```python
from build123d import *

# Parameters (mm, degrees)
F0_R     = 50
F0_R_2   = 40
F1_DEPTH = 15
F2_R     = 50
F2_R_2   = 5
F3_DEPTH = 5
F4_R     = 5
F5_DEPTH = 40


with BuildPart() as f1:
    # F0 (on Front) → F1 (new body)
    with BuildSketch(Plane.XZ):
        Circle(F0_R)
        Circle(F0_R_2, mode=Mode.SUBTRACT)
    extrude(amount=F1_DEPTH)

    # F2 (on face) → F3 (join)
    with BuildSketch(Plane(origin=(0, 0, 0), x_dir=(-1, 0, 0), z_dir=(0, 1, 0))):
        Circle(F2_R)
        Circle(F2_R_2, mode=Mode.SUBTRACT)
    extrude(amount=F3_DEPTH)

    # F4 (on face) → F5 (join)
    with BuildSketch(Plane.XZ.offset(15)):
        with Locations((45, 0)):
            Circle(F4_R)
    extrude(amount=F5_DEPTH)


solid = f1.part
```
Build history of the part. All positions in model axes, mm. A direction names the side the tool comes from. Give positions to 0.01 mm unless a question says otherwise; leave off trailing zeros. Loops run counter-clockwise (first coordinate to the right, second up) from the corner with the lowest first, then second, coordinate; pieces in that order, holes last. Notation, with made-up numbers: (2, 63) - (33, 63) arc R18 ccw to (33, 97) - close; hole circle Ø8 at (31, 68.25). An arc over 180 degrees is marked (long way). Use a Markdown table: item, result.
(1) Band-saw the part on A-A (x = 0). Give the cut face in (y, z), and give its area (3 significant figures).
Taken from the geometry:
| item | result |
|---|---|
| outline | (-15, -50) - (5, -50) - (5, -5) - (0, -5) - (0, -40) - (-15, -40) - close; (-15, 40) - (0, 40) - (0, 5) - (5, 5) - (5, 50) - (-15, 50) - close |
| area | 750 mm2 |
(2) Drop flat-ended pins along their axis: pin 1 Ø6 at (x, y) = (-28.5, -8.5) entering from -Z; pin 2 Ø24 at (x, z) = (-8, 20) entering from -Y; pin 3 Ø5 at (y, z) = (-17, -33.5) entering from -X. Give the stop position or say it passes through.
Taken from the geometry:
| item | result |
|---|---|
| pin 1 | z = -43.01 |
| pin 2 | y = 0 |
| pin 3 | x = -38.42 |
(3) Which spindle directions (+Z, -Z, +X, -X, +Y, -Y) get a long thin tool onto all of the face, cutting with end or side? Do faces 4 (the face through (1, 5, -10)), 5 (the face through (-8, 0, 1)). Say none if no direction does.
Taken from the geometry:
| item | result |
|---|---|
| face 4 | +Z, -Z, +X, -X, +Y |
| face 5 | -Y |
(4) Wall check: line 1 along Z through (x, y) = (0, -5.25); line 2 along Z through (x, y) = (0, 3); line 3 along Y through (x, z) = (-22.5, -32). Give the ranges that are in metal, low to high.
Taken from the geometry:
| item | result |
|---|---|
| line 1 | -50 to -40, 40 to 50 |
| line 2 | -50 to -5, 5 to 50 |
| line 3 | 0 to 5 |
(5) Pull direction X, two halves, no side cores. Call faces 1 (the face through (40, -35, 0)), 2 (the face through (-8.67, -7.4, -39.05)), 3 (the face through (45, -55, 0)): +X half, -X half, draft (parallel to the pull), parting line (faces both ways), or undercut.
Taken from the geometry:
| item | result |
|---|---|
| face 1 | parting line |
| face 2 | undercut |
| face 3 | draft |
(6) Band-saw the part on B-B (z = -11.5). Give the cut face in (x, y).
Taken from the geometry:
| item | result |
|---|---|
| outline | (-48.66, -15) - (-38.31, -15) - (-38.31, 0) - (38.31, 0) - (38.31, -15) - (48.66, -15) - (48.66, 5) - (-48.66, 5) - close |
(7) Band-saw the part on C-C (x = 18). Give the cut face in (y, z).
Taken from the geometry:
| item | result |
|---|---|
| outline | (-15, -46.65) - (5, -46.65) - (5, 46.65) - (-15, 46.65) - (-15, 35.72) - (0, 35.72) - (0, -35.72) - (-15, -35.72) - close |
(8) Band-saw the part on D-D (y = -11.5). Give the cut face in (x, z).
Taken from the geometry:
| item | result |
|---|---|
| outline | circle Ø100 at (0, 0); hole circle Ø80 at (0, 0) |
